```python
from build123d import *

# Parameters (mm, degrees)
CYLINDER004_R             = 4
CYLINDER004_DEPTH         = 10
CYLINDER004_ROLL_ANGLE    = 90
BOX003_W                  = 8
BOX003_H                  = 3
BOX003_DEPTH              = 8
FUSION003_PLACEMENT_ANGLE = 90
CYLINDER005_R             = 4
CYLINDER005_DEPTH         = 10
CYLINDER005_ROLL_ANGLE    = 90
BOX004_W                  = 8
BOX004_H                  = 3
BOX004_DEPTH              = 8
CYLINDER006_R             = 4
CYLINDER006_DEPTH         = 10
CYLINDER006_ROLL_ANGLE    = 90
BOX005_W                  = 8
BOX005_H                  = 3
BOX005_DEPTH              = 8
FUSION005_PLACEMENT_ANGLE = -90
BOX_W                     = 80
BOX_H                     = 8
BOX_DEPTH                 = 8
BOX_PLACEMENT_ANGLE       = 90
CYLINDER_R                = 42
CYLINDER_DEPTH            = 8
THICKNESS_T               = -5
BOX001_W                  = 80
BOX001_H                  = 8
BOX001_DEPTH              = 8
CYLINDER003_R             = 4
CYLINDER003_DEPTH         = 10
CYLINDER003_ROLL_ANGLE    = 90
BOX002_W                  = 8
BOX002_H                  = 3
BOX002_DEPTH              = 8
FUSION002_PLACEMENT_ANGLE = 180


with BuildPart() as cylinder004:
    # Cylinder004 → Cylinder004 (new body)
    with BuildSketch(Plane.XY):
        Circle(CYLINDER004_R)
    extrude(amount=CYLINDER004_DEPTH)


with BuildPart() as cylinder004_1:
    # Cylinder004 roll: moved
    add(cylinder004.part.rotate(Axis((0, 0, 0), (1, 0, 0)), CYLINDER004_ROLL_ANGLE))


with BuildPart() as cylinder004_2:
    # Cylinder004 placement: moved
    add(cylinder004_1.part.moved(Location((0, -41, 4))))


with BuildPart() as obj1:
    # Box003 → Box003 (new body)
    with BuildSketch(Plane(origin=(-4, -43, 0), x_dir=(1, 0, 0), z_dir=(0, 0, 1))):
        with Locations((4, 1.5)):
            Rectangle(BOX003_W, BOX003_H)
    extrude(amount=BOX003_DEPTH)

    # Fusion003: union Cylinder004
    add(cylinder004_2.part)


with BuildPart() as obj1_1:
    # Fusion003 placement: moved
    add(obj1.part.moved(Location((0, 1, 0))).rotate(Axis((0, 1, 0), (0, 0, 1)), FUSION003_PLACEMENT_ANGLE))


with BuildPart() as cylinder005:
    # Cylinder005 → Cylinder005 (new body)
    with BuildSketch(Plane.XY):
        Circle(CYLINDER005_R)
    extrude(amount=CYLINDER005_DEPTH)


with BuildPart() as cylinder005_1:
    # Cylinder005 roll: moved
    add(cylinder005.part.rotate(Axis((0, 0, 0), (1, 0, 0)), CYLINDER005_ROLL_ANGLE))


with BuildPart() as cylinder005_2:
    # Cylinder005 placement: moved
    add(cylinder005_1.part.moved(Location((0, -41, 4))))


with BuildPart() as obj2:
    # Box004 → Box004 (new body)
    with BuildSketch(Plane(origin=(-4, -43, 0), x_dir=(1, 0, 0), z_dir=(0, 0, 1))):
        with Locations((4, 1.5)):
            Rectangle(BOX004_W, BOX004_H)
    extrude(amount=BOX004_DEPTH)

    # Fusion004: union Cylinder005
    add(cylinder005_2.part)


with BuildPart() as cylinder006:
    # Cylinder006 → Cylinder006 (new body)
    with BuildSketch(Plane.XY):
        Circle(CYLINDER006_R)
    extrude(amount=CYLINDER006_DEPTH)


with BuildPart() as cylinder006_1:
    # Cylinder006 roll: moved
    add(cylinder006.part.rotate(Axis((0, 0, 0), (1, 0, 0)), CYLINDER006_ROLL_ANGLE))


with BuildPart() as cylinder006_2:
    # Cylinder006 placement: moved
    add(cylinder006_1.part.moved(Location((0, -41, 4))))


with BuildPart() as obj3:
    # Box005 → Box005 (new body)
    with BuildSketch(Plane(origin=(-4, -43, 0), x_dir=(1, 0, 0), z_dir=(0, 0, 1))):
        with Locations((4, 1.5)):
            Rectangle(BOX005_W, BOX005_H)
    extrude(amount=BOX005_DEPTH)

    # Fusion005: union Cylinder006
    add(cylinder006_2.part)


with BuildPart() as obj3_1:
    # Fusion005 placement: moved
    add(obj3.part.rotate(Axis((0, 0, 0), (0, 0, 1)), FUSION005_PLACEMENT_ANGLE))


with BuildPart() as cube:
    # Box → Box (new body)
    with BuildSketch(Plane.XY):
        with Locations((40, 4)):
            Rectangle(BOX_W, BOX_H)
    extrude(amount=BOX_DEPTH)


with BuildPart() as cube_1:
    # Box placement: moved
    add(cube.part.moved(Location((4, -40, 0))).rotate(Axis((4, -40, 0), (0, 0, 1)), BOX_PLACEMENT_ANGLE))


with BuildPart() as thickness:
    # Cylinder → Cylinder (new body)
    with BuildSketch(Plane.XY):
        Circle(CYLINDER_R)
    extrude(amount=CYLINDER_DEPTH)

    # Thickness
    thickness_openings = [thickness.faces().sort_by_distance(p)[0] for p in [
        (0, 0, 0),
        (0, 0, 8),
    ]]
    offset(amount=THICKNESS_T, openings=thickness_openings)


with BuildPart() as obj4:
    # Box001 → Box001 (new body)
    with BuildSketch(Plane(origin=(-40, -3, 0), x_dir=(1, 0, 0), z_dir=(0, 0, 1))):
        with Locations((40, 4)):
            Rectangle(BOX001_W, BOX001_H)
    extrude(amount=BOX001_DEPTH)

    # Fusion: union Cube, Thickness
    add(cube_1.part)
    add(thickness.part)


with BuildPart() as cylinder003:
    # Cylinder003 → Cylinder003 (new body)
    with BuildSketch(Plane.XY):
        Circle(CYLINDER003_R)
    extrude(amount=CYLINDER003_DEPTH)


with BuildPart() as cylinder003_1:
    # Cylinder003 roll: moved
    add(cylinder003.part.rotate(Axis((0, 0, 0), (1, 0, 0)), CYLINDER003_ROLL_ANGLE))


with BuildPart() as cylinder003_2:
    # Cylinder003 placement: moved
    add(cylinder003_1.part.moved(Location((0, -41, 4))))


with BuildPart() as fusion006:
    # Box002 → Box002 (new body)
    with BuildSketch(Plane(origin=(-4, -43, 0), x_dir=(1, 0, 0), z_dir=(0, 0, 1))):
        with Locations((4, 1.5)):
            Rectangle(BOX002_W, BOX002_H)
    extrude(amount=BOX002_DEPTH)

    # Fusion002: union Cylinder003
    add(cylinder003_2.part)


with BuildPart() as fusion006_1:
    # Fusion002 placement: moved
    add(fusion006.part.rotate(Axis((0, 0, 0), (0, 0, 1)), FUSION002_PLACEMENT_ANGLE))

    # Fusion006: union obj1, obj2, obj3, obj4
    add(obj1_1.part)
    add(obj2.part)
    add(obj3_1.part)
    add(obj4.part)


solid = fusion006_1.part
```
Geometry check sheet. Reference: the model listing, model coordinates, mm. A direction names the side the tool comes from. Round coordinates to 2 decimals unless told otherwise and drop trailing zeros. Order: outer loops, then holes, each group sorted by start corner. A loop starts at its lowest first (then second) coordinate and runs counter-clockwise, first axis right, second up. Notation, with made-up numbers: M 33,67 L 41,67 A18 cw 41,94 Z; hole C -27.5,-15.75 d7. An arc over 180 degrees is marked long. Write item = value, one per line.
Q1. Scan lines: line 1 (X direction, y = 32, z = 1.25); line 2 (Y direction, x = -20, z = 7.75); line 3 (X direction, y = -21.5, z = 1.5). Record each from-to range of solid material in increasing order.
Answer block:
line_1 = -27.2 to -18.57, -4 to 4, 18.57 to 27.2
line_2 = -36.93 to -31.13, -3 to 5, 31.13 to 36.93
line_3 = -36.08 to -30.11, -4 to 4, 30.11 to 36.08
Q2. Depth check by flat-ended pin: pin 1 Ø4 at (y, z) = (-27, 2.5) entering from +X; pin 2 Ø0.6 at (x, z) = (42.5, 3.5) entering from +Y; pin 3 Ø2.5 at (y, z) = (21.5, 5.5) entering from -X. Enter the tip coordinate at first touch or a pass-through.
Answer block:
pin_1 = 33.75
pin_2 = 5
pin_3 = -36.8
Q3. Section check B-B (x = -31.5). Enter the section's corners in (y, z), plus the area to 3 significant figures.
Answer block:
outline = M -27.78,0 L -19.41,0 L -19.41,8 L -27.78,8 Z; M -3,0 L 5,0 L 5,8 L -3,8 Z; M 19.41,0 L 27.78,0 L 27.78,8 L 19.41,8 Z
area = 198 mm^2
Q4. Section check D-D (y = 38.5). Enter the section's corners in (x, z).
Answer block:
outline = M -16.79,0 L 16.79,0 L 16.79,8 L -16.79,8 Z
Q5. Release check for a two-part mould opening along X. For faces 5 (the flat face through (3, -43, 7)), 6 (the cylindrical face through (-0.867, -46.944, 0.095)), 7 (the flat face through (-21, 5, 4)) record: released by +X, released by -X, zero draft, split by the parting line, or undercut.
Answer block:
face_5 = zero draft
face_6 = split by the parting line
face_7 = undercut
Q6. Set-up check for faces 1 (the flat face through (3, 43, 1)), 2 (the flat face through (20, 5, 4)), 3 (the flat face through (-43, -3, 7)), 4 (the flat face through (43, -2, 1)): record each of +Z, -Z, +X, -X, +Y, -Y from which the full face is reachable in a straight line by a thin tool's end or side.
Answer block:
face_1 = -Z, +X, +Y
face_2 = +Z, -Z
face_3 = +Z, -X, -Y
face_4 = -Z, +X, -Y
Q7. Section check C-C (z = 5.75). Give the number of separate pieces and of enclosed holes in the cut face, plus the area to 3 significant figures.
Answer block:
separate_pieces = 1
enclosed_holes = 4
area = 2,620 mm^2
Q8. Section check A-A (y = 26). Enter the section's corners in (x, z).
Answer block:
outline = M -32.98,0 L -26.32,0 L -26.32,8 L -32.98,8 Z; M -4,0 L 4,0 L 4,8 L -4,8 Z; M 26.32,0 L 32.98,0 L 32.98,8 L 26.32,8 Z
